The drawing under review shows one solid part. Ordinate dimensions are in mm from its lowest x, y, z. A direction names the side the tool comes from. Coordinates: 2 decimals unless noted, no trailing zeros. Loops run counter-clockwise (first coordinate to the right, second up) from the corner with the lowest first, then second, coordinate; pieces in that order, holes last. Notation, with made-up numbers: (33.25, 64.5) -> (81.25, 64.5) arc R22 ccw to (81.25, 103.5) -> close; hole circle Ø1 at (51.5, 80). An arc over 180 degrees is marked (long way). Use a Markdown table: item, result.
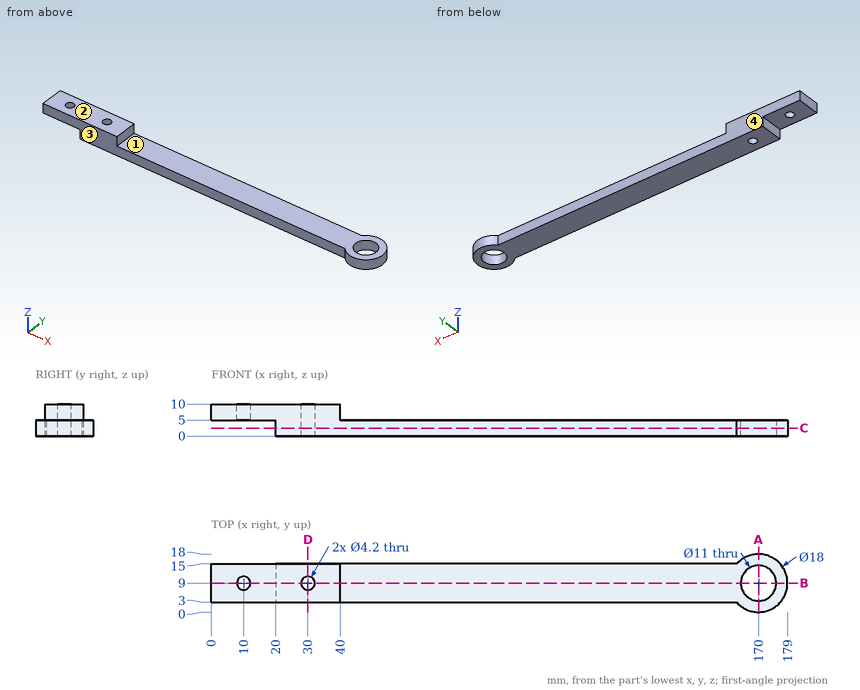
(1) Take a section at A-A on x = 170. Write out the cut boundary in (y, z).
Found:
| item | result |
|---|---|
| outline | (0, 0) -> (3.5, 0) -> (3.5, 5) -> (0, 5) -> close; (14.5, 0) -> (18, 0) -> (18, 5) -> (14.5, 5) -> close |
(2) For the marked faces 1, 2, 3 and 4, list the 3-axis set-ups (+Z, -Z, +X, -X, +Y, -Y) from which the entire face can be reached by the end or side of a thin tool; tool diameter is ignored.
Found:
| item | result |
|---|---|
| face 1 | +Z, +X, +Y, -Y |
| face 2 | +Z, +X, -X, +Y, -Y |
| face 3 | +Z, -Z, -X, -Y |
| face 4 | +Z, -Z, -X, +Y |
(3) Take a section at C-C on z = 2.5. Write out the cut boundary in (x, y).
Found:
| item | result |
|---|---|
| outline | (20, 3) -> (163.29, 3) arc R9 ccw (long way) to (163.29, 15) -> (20, 15) -> close; hole circle Ø4.2 at (30, 9); hole circle Ø11 at (170, 9) |
(4) For pin 1 Ø5.5 at (y, z) = (6.5, 2.5) entering from -X; pin 2 Ø5 at (x, z) = (58, 7) entering from +Y; pin 3 Ø1.5 at (x, z) = (46.5, 7.5) entering from +Y; pin 4 Ø2.5 at (y, z) = (8, 8) entering from +X, all flat-tipped, find the tip position at first contact; note any pin that passes through.
Found:
| item | result |
|---|---|
| pin 1 | stops at x = 0 |
| pin 2 | stops at y = 15 |
| pin 3 | passes through |
| pin 4 | stops at x = 40 |
(5) For line 1 along X through (y, z) = (9, 2.7); line 2 along X through (y, z) = (9, 6.2); line 3 along Y through (x, z) = (30, 3), list the stretches that pass through material, from the lowest coordinate up.
Found:
| item | result |
|---|---|
| line 1 | x = 20 to 27.9, 32.1 to 164.5, 175.5 to 179 |
| line 2 | x = 0 to 7.9, 12.1 to 27.9, 32.1 to 40 |
| line 3 | y = 3 to 6.9, 11.1 to 15 |
(6) Take a section at B-B on y = 9. Write out the cut boundary in (x, z), plus the area to 3 significant figures.
Found:
| item | result |
|---|---|
| outline | (0, 5) -> (7.9, 5) -> (7.9, 10) -> (0, 10) -> close; (12.1, 5) -> (20, 5) -> (20, 0) -> (27.9, 0) -> (27.9, 10) -> (12.1, 10) -> close; (32.1, 0) -> (164.5, 0) -> (164.5, 5) -> (40, 5) -> (40, 10) -> (32.1, 10) -> close; (175.5, 0) -> (179, 0) -> (179, 5) -> (175.5, 5) -> close |
| area | 877 mm^2 |
(7) Take a section at D-D on x = 30. Write out the cut boundary in (y, z).
Found:
| item | result |
|---|---|
| outline | (3, 0) -> (6.9, 0) -> (6.9, 10) -> (3, 10) -> close; (11.1, 0) -> (15, 0) -> (15, 10) -> (11.1, 10) -> close |
